Can you work these out from the model? Positions are in its coordinate system, mm. A direction names the side the tool comes from. Round coordinates to 2 decimals unless told otherwise and drop trailing zeros. Order: outer loops, then holes, each group sorted by start corner. A loop starts at its lowest first (then second) coordinate and runs counter-clockwise, first axis right, second up.
Q1. We'd pull the mould along X, two halves only. Please class faces 3 (the face through (19.9, 65.3, 4.6)), 4 (the face through (24.7, 42.62, 20.88)), 5 (the face through (22.397, 54.653, 24.294)): pulls with the +X half, pulls with the -X half, needs draft (parallel to the pull), parting line crosses it, or undercut.
Q2. Will these pins go through, and if not, where does the flat tip stop? P1, Ø12, axis at y = 57.5, z = 19, coming from the +X side; P2, Ø8, axis at y = 51, z = 8.5, coming from the -X side; P3, Ø12, axis at x = 21.5, y = 24, coming from the +Z side.
Q3. If we section it at B-B (y = 58.5): Please give me the cut outline in (x, z), plus the area to 3 significant figures.
Q4. If I drill on line 1 (Z direction, x = 20, y = 29.5); line 2 (X direction, y = 42, z = 13.5); line 3 (X direction, y = 52, z = 19.5), over which ranges is the centre line in solid material (lowest first)?
Q5. For faces 1 (the face through (22.3, 19.3, 4.8)), 2 (the face through (18.6, 31.98, 24.16)), which set-ups out of +Z, -Z, +X, -X, +Y, -Y let a thin tool reach every point of the face, with its end or its side?
Q6. If we section it at A-A (y = 32): Please give me the cut outline in (x, z).
from build123d import *

# Parameters (mm, degrees)
CYLINDER005_R     = 8.75
CYLINDER005_DEPTH = 40
CYLINDER003_R     = 8.75
CYLINDER003_DEPTH = 40
CYLINDER007_R     = 10.75
CYLINDER007_DEPTH = 40


with BuildPart() as outletextension:
    # Cylinder005 → Cylinder005 (new body)
    with BuildSketch(Plane(origin=(20, 65.3, 13.5), x_dir=(1, 0, 0), z_dir=(0, -1, 0))):
        Circle(CYLINDER005_R)
    extrude(amount=CYLINDER005_DEPTH)


with BuildPart() as inside:
    # Cylinder003 → Cylinder003 (new body)
    with BuildSketch(Plane(origin=(20, 36.3, 13.5), x_dir=(1, 0, 0), z_dir=(0, -1, 0))):
        Circle(CYLINDER003_R)
    extrude(amount=CYLINDER003_DEPTH)

    # Fusion001: union OutletExtension
    add(outletextension.part)


with BuildPart() as housingoutlet:
    # Cylinder007 → Cylinder007 (new body)
    with BuildSketch(Plane(origin=(20, 59.3, 13.5), x_dir=(1, 0, 0), z_dir=(0, -1, 0))):
        Circle(CYLINDER007_R)
    extrude(amount=CYLINDER007_DEPTH)


with BuildPart() as bloweroutletadapter:
    # Cone001 → Cone001 (revolve)
    with BuildSketch(Plane(origin=(20, 65.3, 13.5), x_dir=(-1, 0, 0), z_dir=(0, 0, 1))):
        Polygon((0, 0), (10.92, 0), (11.19, 21), (0, 21), align=None)
    revolve(axis=Axis((20, 65.3, 13.5), (0, -1, 0)))

    # Fusion: union HousingOutlet
    add(housingoutlet.part)

    # Cut: cut inside
    add(inside.part, mode=Mode.SUBTRACT)


solid = bloweroutletadapter.part
Solution:
1. face 3: needs draft
1. face 4: undercut
1. face 5: parting line crosses it
2. P1: stops at x = 31.05
2. P2: stops at x = 8.94
2. P3: stops at z = 24.25
3. outline: circle Ø22.01 at (20, 13.5); hole circle Ø17.5 at (20, 13.5)
3. area: 140 mm2
4. line 1: z = 2.75 to 4.75, 22.25 to 24.25
4. line 2: x = 9.25 to 11.25, 28.75 to 30.75
4. line 3: x = 10.67 to 13.63, 26.37 to 29.33
5. face 1: +Z, -Z, +X, -X, -Y
5. face 2: -Y
6. outline: circle Ø21.5 at (20, 13.5); hole circle Ø17.5 at (20, 13.5)
